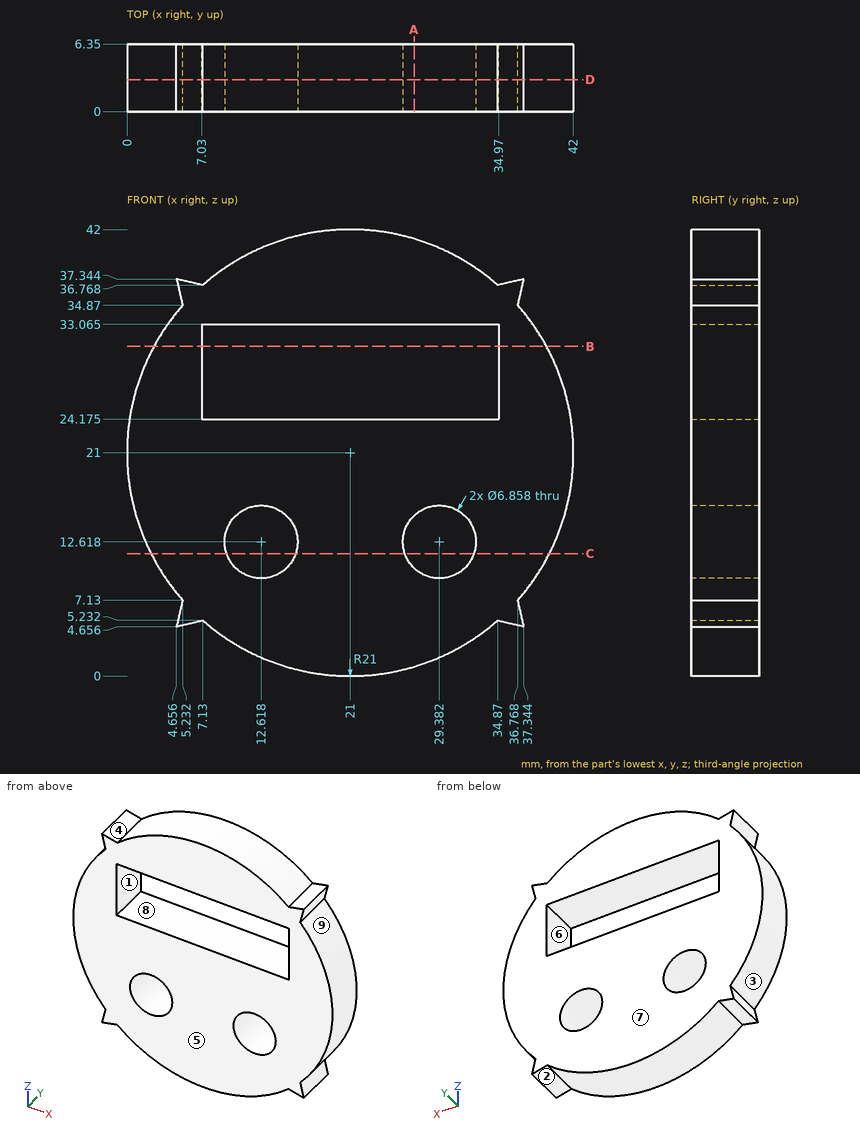
Source: three-view drawing plus pictorial views. Frame: mm from the lowest corner of the part. A direction names the side the tool comes from. Give positions to 0.01 mm unless a question says otherwise; leave off trailing zeros. Loops run counter-clockwise (first coordinate to the right, second up) from the corner with the lowest first, then second, coordinate; pieces in that order, holes last.
1) Reachability of the marked faces 1, 2, 3, 4 and 5 from +Z, -Z, +X, -X, +Y, -Y: full face, straight path, thin tool, end or side. Return the list, or none.
A:
face 1: +Y, -Y
face 2: -Z, +Y, -Y
face 3: -X, +Y, -Y
face 4: +Z, +Y, -Y
face 5: +Z, -Z, +X, -X, -Y
2) Section query C-C on z = 11.5. Return the cut outline in (x, y).
A:
outline: (2.27, 0) - (9.38, 0) - (9.38, 6.35) - (2.27, 6.35) - close; (15.86, 0) - (26.14, 0) - (26.14, 6.35) - (15.86, 6.35) - close; (32.62, 0) - (39.73, 0) - (39.73, 6.35) - (32.62, 6.35) - close
3) Line query: L1, parallel to Z at x = 9.5, y = 1.5 (1 decimal); L2, parallel to X at y = 4, z = 11.5; L3, parallel to Z at x = 13, y = 1.25 (1 decimal). Output: solid intervals per line, ascending.
A:
L1: z = 3.4 to 11.2, 14 to 24.2, 33.1 to 38.6
L2: x = 2.27 to 9.38, 15.86 to 26.14, 32.62 to 39.73
L3: z = 1.6 to 9.2, 16 to 24.2, 33.1 to 40.4
4) Mould query, pull axis X, two halves, no side actions, for the marked faces 6, 7, 8 and 9. Classes: released by +X, released by -X, zero draft, split by the parting line, or undercut.
A:
face 6: undercut
face 7: zero draft
face 8: undercut
face 9: released by +X
5) Contact query for flat-ended pins moving along their axis: pin 1 (5.5 mm diameter, centred on x = 12.618, z = 12.618, fed in from -Y); pin 2 (3 mm diameter, centred on y = 3.5, z = 30, fed in from +X) (1 decimal). Output: stop coordinate, or through.
A:
pin 1: passes through
pin 2: stops at x = 40.6
6) Section query A-A on x = 27. Count the separate pieces of the cut face and the enclosed holes in it, and give its area (3 significant figures).
A:
separate pieces: 3
enclosed holes: 0
area: 168 mm2
7) Section query B-B on z = 31. Return the cut outline in (x, y).
A:
outline: (2.53, 0) - (7.03, 0) - (7.03, 6.35) - (2.53, 6.35) - close; (34.97, 0) - (39.47, 0) - (39.47, 6.35) - (34.97, 6.35) - close
8) Section query D-D on y = 3. Return the cut outline in (x, z) (1 decimal), and give its area (3 significant figures).
A:
outline: (4.7, 4.7) - (7.1, 5.2) arc R21 ccw to (34.9, 5.2) - (37.3, 4.7) - (36.8, 7.1) arc R21 ccw to (36.8, 34.9) - (37.3, 37.3) - (34.9, 36.8) arc R21 ccw to (7.1, 36.8) - (4.7, 37.3) - (5.2, 34.9) arc R21 ccw to (5.2, 7.1) - close; hole (7, 24.2) - (35, 24.2) - (35, 33.1) - (7, 33.1) - close; hole circle Ø6.9 at (12.6, 12.6); hole circle Ø6.9 at (29.4, 12.6)
area: 1,070 mm2
